Build history of the part. All positions in model axes, mm. Face numbers are marked on the shaded views. A direction names the side the tool comes from. Give positions to 0.01 mm unless a question says otherwise; leave off trailing zeros. Order: outer loops, then holes, each group sorted by start corner. A loop starts at its lowest first (then second) coordinate and runs counter-clockwise, first axis right, second up. Notation, with made-up numbers: (-2.5, -31.5) -> (19.5, -31.5) arc R38 cw to (19.5, 6.5) -> close; hole circle Ø4 at (35.5, -30.5). An arc over 180 degrees is marked (long way). One line per question, with ' | ' between items. Start each with the question number.
(1) Cut at C-C (x = -24.5). Give the cut face in (y, z).
(2) Pull direction X, two halves, no side cores. Call the marked faces 1, 2, 3 and 4: +X half, -X half, draft (parallel to the pull), parting line (faces both ways), or undercut.
(3) Which spindle directions (+Z, -Z, +X, -X, +Y, -Y) get a long thin tool onto all of the face, cutting with end or side? Do the marked faces 5, 6, 7, 8 and 9. Say none if no direction does.
(4) Drill centre lines: L1, parallel to Z at x = 0, y = 48.5; L2, parallel to Z at x = 20.5, y = 14.5. Where is each one in solid material? Low to high. Write a range as from..to.
(5) Cut at A-A (x = 0). Give the cut face in (y, z).
(6) Pin check, flat tips, straight feed: pin 1 Ø6 at (y, z) = (38, -14.5) entering from +X; pin 2 Ø3 at (x, z) = (15.5, 6.5) entering from -Y; pin 3 Ø3 at (x, y) = (15.5, 64) entering from -Z. Stop position of each tip, or through.
(7) Cut at B-B (z = 0). Give the cut face in (x, y), then the cut area to 3 significant figures.
(8) Cut at D-D (y = 42.5). Give the cut face in (x, z), then the cut area to 3 significant figures.
from build123d import *

# Parameters (mm, degrees)
SKETCH2_W               = 60
SKETCH2_H               = 60
BOSS_EXTRUDE2_DEPTH     = 32
SKETCH3_W               = 35
SKETCH3_H               = 20
CUT_EXTRUDE1_DEPTH      = 60
SKETCH4_W               = 35
SKETCH4_H               = 20
CUT_EXTRUDE2_DEPTH      = 61
SKETCH5_R               = 17.5
BOSS_EXTRUDE3_DEPTH     = 64
SKETCH6_R               = 10
CUT_EXTRUDE3_DEPTH      = 1
CUT_EXTRUDE3_DEPTH_BACK = 97


with BuildPart() as part:
    # Sketch2 → Boss-Extrude2 (new body)
    with BuildSketch(Plane(origin=(0, 0, 0), x_dir=(1, 0, 0), z_dir=(0, 1, 0))):
        Rectangle(SKETCH2_W, SKETCH2_H)
    extrude(amount=BOSS_EXTRUDE2_DEPTH)

    # Sketch3 → Cut-Extrude1 (cut)
    with BuildSketch(Plane.XY.offset(30)):
        with Locations((0, 10)):
            Rectangle(SKETCH3_W, SKETCH3_H)
    extrude(amount=-CUT_EXTRUDE1_DEPTH, mode=Mode.SUBTRACT)

    # Sketch4 → Cut-Extrude2 (cut, through all)
    with BuildSketch(Plane(origin=(30, 0, 0), x_dir=(0, 0, -1), z_dir=(1, 0, 0))):
        with Locations((0, 10)):
            Rectangle(SKETCH4_W, SKETCH4_H)
    extrude(amount=-CUT_EXTRUDE2_DEPTH, mode=Mode.SUBTRACT)

    # Sketch5 → Boss-Extrude3 (add)
    with BuildSketch(Plane(origin=(0, 32, 0), x_dir=(1, 0, 0), z_dir=(0, 1, 0))):
        Circle(SKETCH5_R)
    extrude(amount=BOSS_EXTRUDE3_DEPTH)

    # Sketch6 → Cut-Extrude3 (cut, two sides)
    with BuildSketch(Plane(origin=(0, 96, 0), x_dir=(1, 0, 0), z_dir=(0, 1, 0))) as cut_extrude3_sk:
        Circle(SKETCH6_R)
    extrude(amount=CUT_EXTRUDE3_DEPTH, mode=Mode.SUBTRACT)
    extrude(cut_extrude3_sk.sketch, amount=-CUT_EXTRUDE3_DEPTH_BACK, mode=Mode.SUBTRACT)


solid = part.part
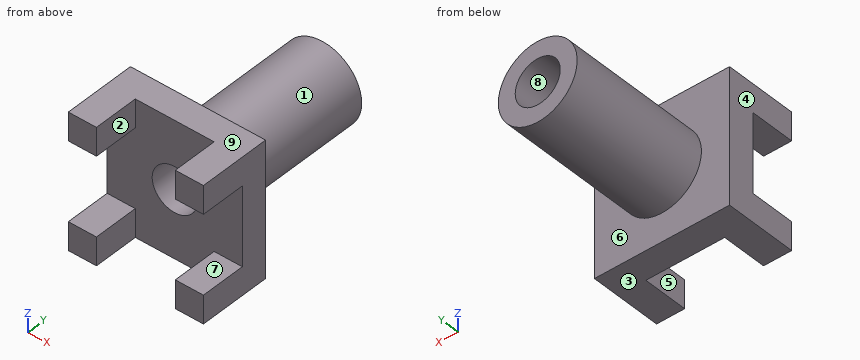
Result set:
1) outline: (0, -30) -> (32, -30) -> (32, 30) -> (0, 30) -> (0, 17.5) -> (20, 17.5) -> (20, -17.5) -> (0, -17.5) -> close
2) face 1: parting line | face 2: undercut | face 3: draft | face 4: -X half
3) face 5: +Z, -Z, -Y | face 6: +Y | face 7: +X, -X, -Y | face 8: +Y, -Y | face 9: +Z, +X, -X, +Y, -Y
4) L1: z = -17.5..-10, 10..17.5 | L2: z = -30..-17.5, 17.5..30
5) outline: (20, -30) -> (32, -30) -> (32, -17.5) -> (96, -17.5) -> (96, -10) -> (20, -10) -> close; (20, 10) -> (96, 10) -> (96, 17.5) -> (32, 17.5) -> (32, 30) -> (20, 30) -> close
6) pin 1: stops at x = 13.19 | pin 2: stops at y = 20 | pin 3: stops at z = -10.5
7) outline: (-30, 20) -> (-10, 20) -> (-10, 96) -> (-17.5, 96) -> (-17.5, 32) -> (-30, 32) -> close; (10, 20) -> (30, 20) -> (30, 32) -> (17.5, 32) -> (17.5, 96) -> (10, 96) -> close | area: 1,440 mm2
8) outline: circle Ø35 at (0, 0); hole circle Ø20 at (0, 0) | area: 648 mm2
